```python
from build123d import *

# Parameters (mm, degrees)
BOSS_EXTRUDE1_DEPTH = 20
SKETCH2_R           = 4
CUT_EXTRUDE1_DEPTH  = 30
SKETCH3_R           = 4
CUT_EXTRUDE2_DEPTH  = 30
CUT_EXTRUDE3_DEPTH  = 87


with BuildPart() as part:
    # Sketch1 → Boss-Extrude1 (new body)
    with BuildSketch(Plane.XY):
        Polygon((0, 177), (0, 167), (30, 167), (70, 116), (70, 56), (30, 5), (0, 5), (0, -5), (34.865710136, -5), (80, 52.546219577), (80, 119.453780423), (34.865710136, 177), align=None)
    extrude(amount=BOSS_EXTRUDE1_DEPTH)

    # Sketch2 → Cut-Extrude1 (cut)
    with BuildSketch(Plane.ZY):
        with Locations(Location((10, 172, 0), (0, 0, 270))):
            Circle(SKETCH2_R)
        with Locations(Location((10, 0, 0), (0, 0, 90))):
            Circle(SKETCH2_R)
    extrude(amount=-CUT_EXTRUDE1_DEPTH, mode=Mode.SUBTRACT)

    # Sketch3 → Cut-Extrude2 (cut)
    with BuildSketch(Plane(origin=(80, 0, 0), x_dir=(0, 0, -1), z_dir=(1, 0, 0))):
        with Locations((-10, 102.726890212)):
            Circle(SKETCH3_R)
        with Locations((-10, 69.273109788)):
            Circle(SKETCH3_R)
    extrude(amount=-CUT_EXTRUDE2_DEPTH, mode=Mode.SUBTRACT)

    # Sketch4 → Cut-Extrude3 (cut)
    with BuildSketch(Plane(origin=(80, 0, 0), x_dir=(0, 0, -1), z_dir=(1, 0, 0))):
        with BuildLine():
            Line((-14, 163), (-6, 163))
            ThreePointArc((-6, 163), (-4.585786438, 162.414213562), (-4, 161))
            Line((-4, 161), (-4, 125.453780423))
            ThreePointArc((-4, 125.453780423), (-4.585786438, 124.039566861), (-6, 123.453780423))
            Line((-6, 123.453780423), (-14, 123.453780423))
            ThreePointArc((-14, 123.453780423), (-15.414213562, 124.039566861), (-16, 125.453780423))
            Line((-16, 125.453780423), (-16, 161))
            ThreePointArc((-16, 161), (-15.414213562, 162.414213562), (-14, 163))
        make_face()
        with BuildLine():
            Line((-14, 48.546219577), (-6, 48.546219577))
            ThreePointArc((-6, 48.546219577), (-4.585786438, 47.960433139), (-4, 46.546219577))
            Line((-4, 46.546219577), (-4, 11))
            ThreePointArc((-4, 11), (-4.585786438, 9.585786438), (-6, 9))
            Line((-6, 9), (-14, 9))
            ThreePointArc((-14, 9), (-15.414213562, 9.585786438), (-16, 11))
            Line((-16, 11), (-16, 46.546219577))
            ThreePointArc((-16, 46.546219577), (-15.414213562, 47.960433139), (-14, 48.546219577))
        make_face()
    extrude(amount=-CUT_EXTRUDE3_DEPTH, mode=Mode.SUBTRACT)


solid = part.part
```
Design review of the part built by this model. Coordinates are the model's own, in mm. A direction names the side the tool comes from. Coordinates: 2 decimals unless noted, no trailing zeros. Loops run counter-clockwise (first coordinate to the right, second up) from the corner with the lowest first, then second, coordinate; pieces in that order, holes last. Notation, with made-up numbers: (-27, 79) -> (-20, 79) arc R24 ccw to (-20, 89) -> close; hole circle Ø10 at (-12, 87). An arc over 180 degrees is marked (long way). Answer as a JSON object with one key per item and string values.
Q1. Tool access review of faces 1 (the cylindrical face through (14.79, -0.867, 13.905)), 2 (the flat face through (57.117, 23.37, 3.193)), 3 (the flat face through (49.72, 141.86, 3.19)), 4 (the flat face through (55, 29, 16)), 5 (the flat face through (80, 86, 10)): name each direction out of +Z, -Z, +X, -X, +Y, -Y from which nothing blocks a thin tool from reaching the whole face with its end or side.
Answer block:
{"face 1": "-X", "face 2": "+Z, -Z, +X, -Y", "face 3": "+Z, -Z, -X", "face 4": "+X, -X", "face 5": "+Z, -Z, +X, +Y, -Y"}
Q2. Take a section at C-C on y = 26. Give the boundary of the cut face in (x, z), plus the area to 3 significant figures.
Answer block:
{"outline": "(46.47, 0) -> (59.18, 0) -> (59.18, 4) -> (46.47, 4) -> close; (46.47, 16) -> (59.18, 16) -> (59.18, 20) -> (46.47, 20) -> close", "area": "102 mm^2"}
Q3. Take a section at A-A on x = 24.5. Give the boundary of the cut face in (y, z).
Answer block:
{"outline": "(-5, 0) -> (5, 0) -> (5, 20) -> (-5, 20) -> close; (167, 0) -> (177, 0) -> (177, 20) -> (167, 20) -> close; hole circle Ø8 at (0, 10); hole circle Ø8 at (172, 10)"}
Q4. Clearance check with flat-ended pins moving along their axes: pin 1 Ø1.5 at (y, z) = (24, 4.5) entering from +X; pin 2 Ø2.5 at (x, z) = (39.5, 9.5) entering from -Y; pin 3 Ø6.5 at (x, z) = (38.5, 11.5) entering from +Y; pin 4 Ø10.5 at (y, z) = (0, 10) entering from -X. State where each tip first meets the part, or that it passes through.
Answer block:
{"pin 1": "stops at x = 58.05", "pin 2": "stops at y = -0.69", "pin 3": "stops at y = 176.51", "pin 4": "stops at x = 0"}
Q5. The part is to be moulded in two halves that separate along Y. For faces 6 (the flat face through (40, 163, 10)), 7 (the flat face through (71, 48.546, 10)), 8 (the flat face through (71, 123.454, 10)), 9 (the cylindrical face through (14.79, 168.185, 11.201)), say which applies: +Y half, -Y half, draft (parallel to the pull), parting line (faces both ways), or undercut.
Answer block:
{"face 6": "undercut", "face 7": "-Y half", "face 8": "+Y half", "face 9": "undercut"}
Q6. Take a section at D-D on x = 55. Give the boundary of the cut face in (y, z) (3 decimals).
Answer block:
{"outline": "(20.671, 0) -> (36.875, 0) -> (36.875, 4) -> (20.671, 4) -> close; (20.671, 16) -> (36.875, 16) -> (36.875, 20) -> (20.671, 20) -> close; (135.125, 0) -> (151.329, 0) -> (151.329, 4) -> (135.125, 4) -> close; (135.125, 16) -> (151.329, 16) -> (151.329, 20) -> (135.125, 20) -> close"}
Q7. To check wall thickness, follow L1, parallel to Y at x = 76, z = 10; L2, parallel to Z at x = 65, y = 45.5; L3, parallel to Y at x = 6, z = 7.75. State the ranges of each line that lie inside material, in increasing order.
Answer block:
{"L1": "y = 48.55 to 65.27, 73.27 to 98.73, 106.73 to 123.45", "L2": "z = 0 to 4, 16 to 20", "L3": "y = -5 to -3.31, 3.31 to 5, 167 to 168.69, 175.31 to 177"}
Q8. Take a section at B-B on z = 2.25. Give the boundary of the cut face in (x, y), plus the area to 3 significant figures.
Answer block:
{"outline": "(0, -5) -> (34.87, -5) -> (80, 52.55) -> (80, 119.45) -> (34.87, 177) -> (0, 177) -> (0, 167) -> (30, 167) -> (70, 116) -> (70, 56) -> (30, 5) -> (0, 5) -> close", "area": "2,660 mm^2"}
